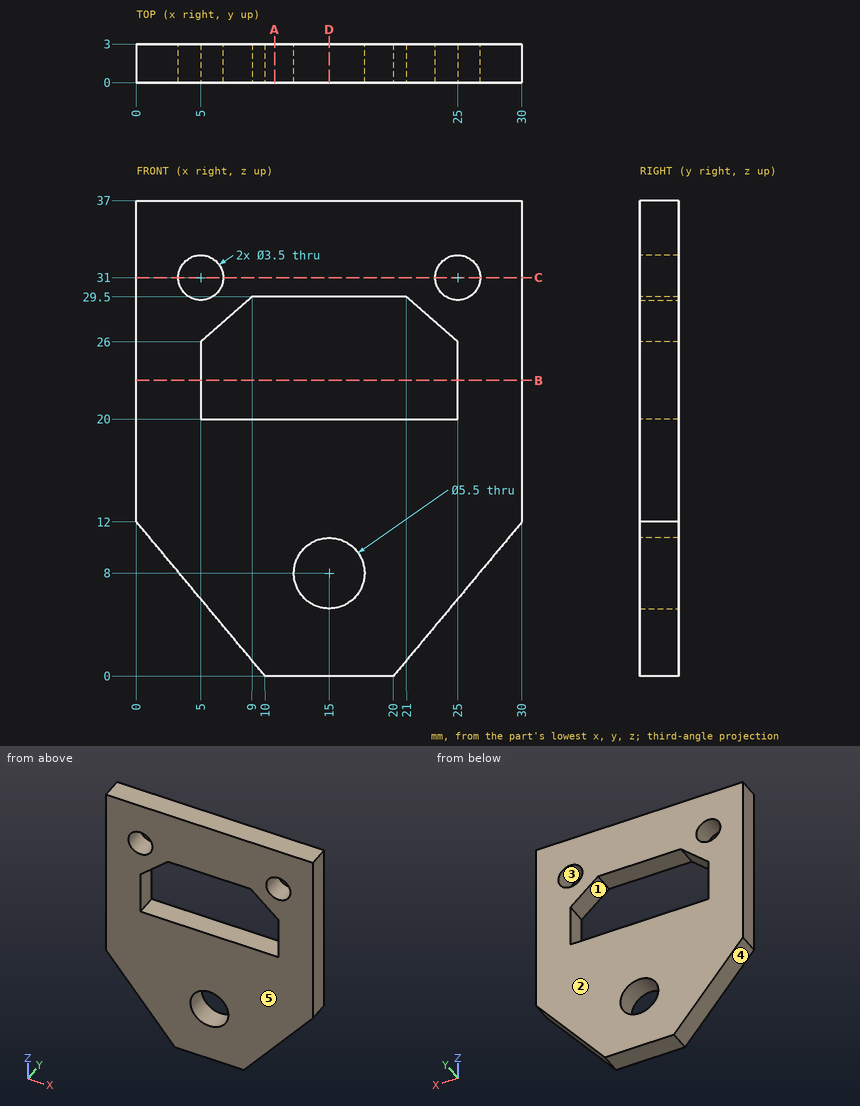
Design review of the part shown in the three views and the two pictorial views. Dimensions are in mm from the part's minimum x, y and z. A direction names the side the tool comes from. Round coordinates to 2 decimals unless told otherwise and drop trailing zeros. Write each loop counter-clockwise with the first axis right and the second up, starting at its lowest first coordinate (ties: lowest second). Pieces come first, ordered by that corner, then holes.
Item 1: We need section C-C on z = 31. Write out the cut boundary in (x, y), and give its area (3 significant figures).
Item 2: We need section D-D on x = 15. Write out the cut boundary in (y, z), and give its area (3 significant figures).
Item 3: For the marked faces 1 and 2, list the 3-axis set-ups (+Z, -Z, +X, -X, +Y, -Y) from which the entire face can be reached by the end or side of a thin tool; tool diameter is ignored.
Item 4: Clearance check with a flat-ended pin moving along its axis: pin 1 Ø3 at (x, z) = (5, 31) entering from +Y. State where the tip first meets the part, or that it passes through.
Item 5: We need section B-B on z = 23. Write out the cut boundary in (x, y), and give its area (3 significant figures).
Item 6: For probe 1 along X at (y, z) = (1.4, 31); probe 2 along Z at (x, y) = (18.25, 1.5); probe 3 along X at (y, z) = (2.35, 26), list the stretches that pass through material, from the lowest coordinate up.
Item 7: The part is to be moulded in two halves that separate along Z. For the marked faces 3, 4 and 5, say which applies: +Z half, -Z half, draft (parallel to the pull), parting line (faces both ways), or undercut.
Item 8: We need section A-A on x = 10.75. Write out the cut boundary in (y, z).
Returned:
1. outline: (0, 0) - (3.25, 0) - (3.25, 3) - (0, 3) - close; (6.75, 0) - (23.25, 0) - (23.25, 3) - (6.75, 3) - close; (26.75, 0) - (30, 0) - (30, 3) - (26.75, 3) - close
1. area: 69.0 mm2
2. outline: (0, 0) - (3, 0) - (3, 5.25) - (0, 5.25) - close; (0, 10.75) - (3, 10.75) - (3, 20) - (0, 20) - close; (0, 29.5) - (3, 29.5) - (3, 37) - (0, 37) - close
2. area: 66.0 mm2
3. face 1: +Y, -Y
3. face 2: +Z, -Z, +X, -X, +Y
4. pin 1: passes through
5. outline: (0, 0) - (5, 0) - (5, 3) - (0, 3) - close; (25, 0) - (30, 0) - (30, 3) - (25, 3) - close
5. area: 30.0 mm2
6. probe 1: x = 0 to 3.25, 6.75 to 23.25, 26.75 to 30
6. probe 2: z = 0 to 20, 29.5 to 37
6. probe 3: x = 0 to 5, 25 to 30
7. face 3: undercut
7. face 4: -Z half
7. face 5: draft
8. outline: (0, 0) - (3, 0) - (3, 20) - (0, 20) - close; (0, 29.5) - (3, 29.5) - (3, 37) - (0, 37) - close
